Read the model definition and answer for the solid it produces. Units are mm, in the model's axes. A direction names the side the tool comes from. Give positions to 0.01 mm unless a question says otherwise; leave off trailing zeros. Write each loop counter-clockwise with the first axis right and the second up, starting at its lowest first coordinate (ties: lowest second). Pieces come first, ordered by that corner, then holes. Notation, with made-up numbers: (16, 41.5) -> (36, 41.5) arc R31 cw to (36, 71.5) -> close; hole circle Ø2 at (75.25, 36). An arc over 180 degrees is marked (long way). Answer as CSV lines item,"result". Start each with the question number.
1. The part is cut by section A-A, the plane y = 33.5. Determine the outline of the cut face in (x, z).
2. The part is cut by section C-C, the plane x = 17. Determine the outline of the cut face in (y, z), and give its area (3 significant figures).
3. The part is cut by section B-B, the plane z = 21. Determine the outline of the cut face in (x, y), and give its area (3 significant figures).
4. Given pin 1 (12 mm diameter, centred on y = 30, z = 27.5, fed in from -X); pin 2 (1.5 mm diameter, centred on x = 17, z = 33.5, fed in from -Y); pin 3 (8 mm diameter, centred on x = 35, z = 7.5, fed in from -Y), each flat-ended and moving along its own axis, determine where each tip first touches the part or whether it passes through.
5. Find the intervals of material crossed by line 1 (Y direction, x = 12, z = 36); line 2 (Y direction, x = 36.5, z = 16); line 3 (Z direction, x = 10, y = 35.5), in increasing order.
6. A tool of negligible diameter and unlimited length cuts with its end or side. For faces 1 (the flat face through (5.7, 11.4, 28.6)), 2 (the flat face through (40, 29, 11)), from which of +Z, -Z, +X, -X, +Y, -Y can it reach the whole face along a straight path? Write none if from no direction.
from build123d import *

# Parameters (mm, degrees)
F1_DEPTH = 40
F3_DEPTH = 40
F6_DEPTH = 16.3309316186


with BuildPart() as f1:
    # F0 (on Right) → F1 (new body)
    with BuildSketch(Plane.YZ):
        Polygon((40, 40), (0, 0), (40, 0), align=None)
    extrude(amount=F1_DEPTH)

    # F2 (on face) → F3 (join)
    with BuildSketch(Plane(origin=(0, 0, 0), x_dir=(1, 0, 0), z_dir=(0, 0, -1))):
        Polygon((20, -40), (0, 0), (0, -40), align=None)
    extrude(amount=-F3_DEPTH)

    # F5 (on 3pt) → F6 (cut, through all)
    with BuildSketch(Plane(origin=(-13.3333333333, 6.6666666667, 6.6666666667), x_dir=(0.3651483717, 0.9128709292, -0.1825741858), z_dir=(0.8164965809, -0.4082482905, -0.4082482905))):
        Polygon((36.514837167, 0), (36.514837167, 44.72135955), (-7.3029674334, 35.77708764), align=None)
    extrude(amount=-F6_DEPTH, mode=Mode.SUBTRACT)


solid = f1.part
Results found:
1,outline,"(0, 0) -> (40, 0) -> (40, 33.5) -> (16.75, 33.5) -> (16.75, 40) -> (0, 6.5) -> close"
2,outline,"(0, 0) -> (40, 0) -> (40, 34) -> (34, 40) -> (34, 34) -> close"
2,area,"800 mm²"
3,outline,"(0, 0) -> (10.5, 21) -> (40, 21) -> (40, 40) -> (10.5, 40) -> (0, 19) -> close"
3,area,"760 mm²"
4,pin 1,"stops at x = 4.51"
4,pin 2,"stops at y = 32.5"
4,pin 3,"stops at y = 3.5"
5,line 1,"y = 24 to 28"
5,line 2,"y = 16 to 40"
5,line 3,"z = 0 to 24.5"
6,face 1,"+Z, +X, -Y"
6,face 2,"+Z, -Z, +X, +Y, -Y"
